from build123d import *

# Parameters (mm, degrees)
F1_DEPTH = 16
F2_W     = 14.5
F2_H     = 11
F3_DEPTH = 15
F5_DEPTH = 23.501
F7_D     = 4.2
F9_D     = 4.2
F10_SIZE = 3


with BuildPart() as f1:
    # F0 (on Right) → F1 (new body)
    with BuildSketch(Plane.YZ):
        with BuildLine():
            ThreePointArc((-7.0647009845, 6.5), (9.6, 0), (-7.0647009845, -6.5))
            Line((-7.0647009845, -6.5), (-12, -6.5))
            Line((-12, -6.5), (-12, -27))
            Line((-12, -27), (20, -27))
            Line((20, -27), (20, 20))
            Line((20, 20), (-12, 20))
            Line((-12, 20), (-12, 6.5))
            Line((-12, 6.5), (-7.0647009845, 6.5))
        make_face()
    extrude(amount=F1_DEPTH)

    # F2 (on face) → F3 (join)
    with BuildSketch(Plane.YZ.offset(16)):
        with Locations((3.75, -21.5)):
            Rectangle(F2_W, F2_H)
    extrude(amount=F3_DEPTH)

    # F4 (on face) → F5 (cut, through all)
    with BuildSketch(Plane.XZ.offset(3.5)):
        Polygon((29.8309389108, -16), (31, -21.5), (31, -16), align=None)
    extrude(amount=-F5_DEPTH, mode=Mode.SUBTRACT)

    # F7 (through all)
    with Locations(Plane(origin=(0, 11, 0), x_dir=(-1, 0, 0), z_dir=(0, 1, 0))):
        with Locations((-26, -21.5)):
            Hole(F7_D / 2)

    # F9 (through all)
    with Locations(Plane(origin=(0, 20, 0), x_dir=(-1, 0, 0), z_dir=(0, 1, 0))):
        with Locations((-8, 0)):
            Hole(F9_D / 2)

    # F10
    f10_edges = [f1.edges().sort_by_distance(p)[0] for p in [
        (8, -12, 6.5),
        (8, -12, -6.5),
    ]]
    chamfer(f10_edges, length=F10_SIZE)


solid = f1.part
Design review of the part built by this model. Coordinates are the model's own, in mm. A direction names the side the tool comes from. Give positions to 0.01 mm unless a question says otherwise; leave off trailing zeros. Order: outer loops, then holes, each group sorted by start corner. A loop starts at its lowest first (then second) coordinate and runs counter-clockwise, first axis right, second up. Notation, with made-up numbers: (22.25, 46) - (77.25, 46) arc R15 cw to (77.25, 66) - close; hole circle Ø3 at (-9.5, -5). An arc over 180 degrees is marked (long way). Use CSV: the item, a comma, the result in double quotes. Start each with the question number.
Q1. Take a section at C-C (z = 0). State the section outline as (x, y) points.
Q2. For line 1 (Z direction, x = 4, y = 0); line 2 (Z direction, x = 26, y = 2.5); line 3 (Y direction, x = 4.5, z = 0), list the stretches that pass through material, from the lowest coordinate up.
Q3. Draft analysis for pull direction X (two halves, no side actions). For faces 5 (the face through (5.9, 14.61, 0.09)), 6 (the face through (30.407, 3.649, -18.712)), 7 (the face through (7.9, -10.5, 8)), state which applies: pulls with the +X half, pulls with the -X half, needs draft (parallel to the pull), parting line crosses it, or undercut.
Q4. Machinability: for faces 1 (the face through (23, -3.5, -22)), 2 (the face through (23, 11, -22)), 3 (the face through (23, 4, -16)), 4 (the face through (7.9, -10.5, -8)), which of the approach directions +Z, -Z, +X, -X, +Y, -Y give a long, thin tool a straight path to every point of the face, cutting with its end or side? Answer none if there is none.
Q5. Take a section at D-D (x = 14). State the section outline as (y, z) points, and give its area (3 significant figures).
Q6. Take a section at A-A (x = 26). State the section outline as (y, z) points.
Q7. Take a section at B-B (y = 3.5). State the section outline as (x, z) points.
Q8. For P1, Ø2.5, axis at x = 8, z = 0, coming from the +Y side; P2, Ø10, axis at x = 16.5, y = 14.5, coming from the -Z side; P3, Ø5.5, axis at x = 26, z = -24, coming from the +Y side; P4, Ø9, axis at x = 26, z = -23.5, coming from the -Y side, all flat-tipped, find the tip position at first contact; note any pin that passes through.
Calculated:
1,outline,"(0, 9.6) - (5.9, 9.6) - (5.9, 20) - (0, 20) - close; (10.1, 9.6) - (16, 9.6) - (16, 20) - (10.1, 20) - close"
2,line 1,"z = -27 to -9.6, 9.6 to 20"
2,line 2,"z = -27 to -23.6, -19.4 to -16"
2,line 3,"y = 9.6 to 20"
3,face 5,"undercut"
3,face 6,"pulls with the +X half"
3,face 7,"needs draft"
4,face 1,"+Z, -Z, +X, -Y"
4,face 2,"+Z, -Z, +X, +Y"
4,face 3,"+Z, +X, +Y, -Y"
4,face 4,"+X, -X, -Y"
5,outline,"(-12, -27) - (20, -27) - (20, 20) - (-12, 20) - (-12, 9.5) - (-9, 6.5) - (-7.06, 6.5) arc R9.6 cw (long way) to (-7.06, -6.5) - (-9, -6.5) - (-12, -9.5) - close"
5,area,"1,160 mm²"
6,outline,"(-3.5, -27) - (11, -27) - (11, -23.6) - (-3.5, -23.6) - close; (-3.5, -19.4) - (11, -19.4) - (11, -16) - (-3.5, -16) - close"
7,outline,"(0, -27) - (31, -27) - (31, -21.5) - (29.83, -16) - (16, -16) - (16, -8.94) - (0, -8.94) - close; (0, 8.94) - (16, 8.94) - (16, 20) - (0, 20) - close; hole circle Ø4.2 at (26, -21.5)"
8,P1,"passes through"
8,P2,"stops at z = -27"
8,P3,"stops at y = 11"
8,P4,"stops at y = -3.5"
